Read the model definition and answer for the solid it produces. Units are mm, in the model's axes. Face numbers are marked on the shaded views. A direction names the side the tool comes from. Give positions to 0.01 mm unless a question says otherwise; leave off trailing zeros. Order: outer loops, then holes, each group sorted by start corner. A loop starts at its lowest first (then second) coordinate and runs counter-clockwise, first axis right, second up. Notation, with made-up numbers: (74, -7) -> (85, -7) arc R23 cw to (85, 29) -> close; hole circle Ø4 at (-13, -2.75). An arc over 180 degrees is marked (long way). Answer as CSV lines item,"result". Start each with the question number.
1) Find section A-A (x = 24). Determine the outline of the cut face in (y, z).
2) Find section D-D (x = 20.5). Determine the outline of the cut face in (y, z).
3) For the marked faces 1, 2 and 3, determine the directions among +Z, -Z, +X, -X, +Y, -Y from which every point of the face is accessible in a straight line to the end or side of a thin tool.
4) Straight lines are drawn through the part: L1, parallel to X at y = 5, z = 13.7; L2, parallel to Z at x = 25.25, y = 3.5; L3, parallel to X at y = 4, z = 13. For each, find the intervals that lie inside material, in ascending order. Write a range as from..to.
5) Flat-ended cylindrical pins translate along their axes: pin 1 Ø3 at (y, z) = (5, 11.5) entering from -X; pin 2 Ø8 at (x, z) = (20.5, 11) entering from +Y; pin 3 Ø3 at (y, z) = (1.5, 6.5) entering from -X. Find the tip coordinate at first contact, or state that the pin passes through.
6) The mould has two halves that part along X. Classify the marked faces 4, 5 and 6: +X half, -X half, draft (parallel to the pull), parting line (faces both ways), or undercut.
Autodesk Fusion 360 part; units mm, degrees
sketch "Skizze1" plane through (0, 0, 0) normal (0, 0, 1) x (1, 0, 0)
  line L0 (0, 0) -> (15, 0)
  line L1 (15, 0) -> (15, 10)
  line L2 (15, 10) -> (0, 10)
  line L3 (0, 10) -> (0, 0)
  dimension "d1" = 15
  dimension "d2" = 10
extrude "Extrusion1" add sketch "Skizze1" along normal blind 12.9
sketch "Skizze2" plane through (0, 0, 12.9) normal (0, 0, 1) x (-1, 0, 0)
  line L0 (0, -10) -> (0, 0)
  line L1 (0, 0) -> (-15, 0)
  line L2 (-15, 0) -> (-15, -10)
  line L3 (-15, -10) -> (0, -10)
  circle A0 centre (-24, -5) radius 1.15
  line L4 (0, -10) -> (-15, -10)
  line L5 (-15, -10) -> (-29, -9)
  line L6 (-29, -9) -> (-29, -1)
  line L7 (-29, -1) -> (-15, 0)
  dimension "Bohrung" = 2.3
  dimension "d8" = 8
  dimension "d9" = 1
  dimension "d12" = 5
  dimension "d21" = 4
  dimension "d22" = 10
extrude "Extrusion2" add sketch "Skizze2" along normal blind 1.6
fillet "Abrundung1" radius 4 2 edges at (29, 9, 13.7) (29, 1, 13.7)
fillet "Abrundung2" radius 5 4 edges at (15, 10, 6.45) (15, 0, 6.45) (0, 0, 7.25) (0, 10, 7.25)
fillet "Abrundung3" radius 1 1 edges at (15, 5, 12.9)
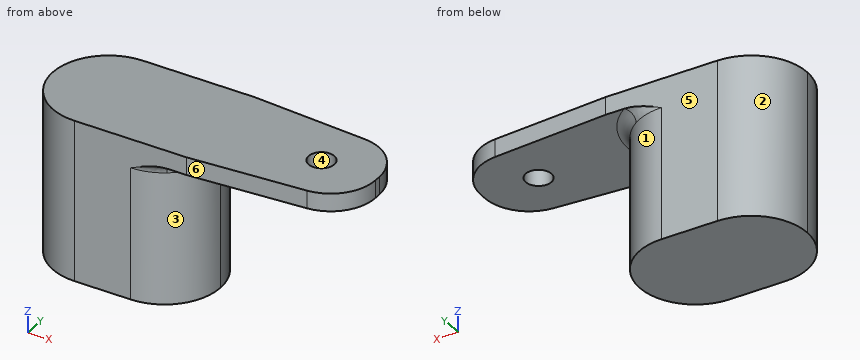
Findings below:
1,outline,"(0.64, 12.9) -> (3.85, 12.9) -> (3.85, 14.5) -> (0.64, 14.5) -> close; (6.15, 12.9) -> (9.36, 12.9) -> (9.36, 14.5) -> (6.15, 14.5) -> close"
2,outline,"(0.39, 12.9) -> (9.61, 12.9) -> (9.61, 14.5) -> (0.39, 14.5) -> close"
3,face 1,"-Z, +X, +Y"
3,face 2,"+Z, -Z, -X, +Y"
3,face 3,"-Z, +X, -Y"
4,L1,"0..22.85, 25.15..29"
4,L2,"12.9..14.5"
4,L3,"0.1..23.43, 24.57..28.93"
5,pin 1,"x = 0"
5,pin 2,"y = 9.86"
5,pin 3,"x = 0.42"
6,face 4,"undercut"
6,face 5,"draft"
6,face 6,"+X half"
